Input: dimensioned drawing with shaded views. Units: mm. Origin: part minimum x, y, z. Give positions to 0.01 mm unless a question says otherwise; leave off trailing zeros. Loops run counter-clockwise (first coordinate to the right, second up) from the corner with the lowest first, then second, coordinate; pieces in that order, holes last.
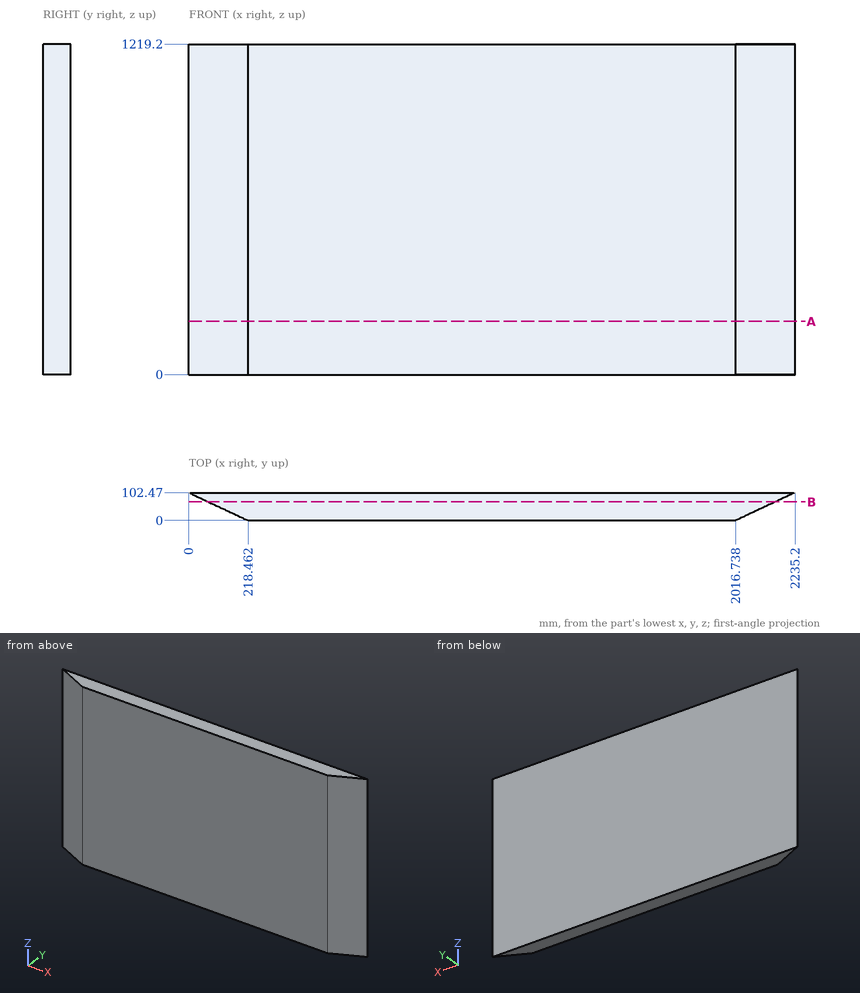
Item 1: Section query B-B on y = 68.5. Return loops of the section in (x, z).
Values follow:
outline: (72.42, 0) - (2162.78, 0) - (2162.78, 1219.2) - (72.42, 1219.2) - close
Item 2: Ray query, probe 1 along X at (y, z) = (5, 685); probe 2 along X at (y, z) = (37, 176); probe 3 along Y at (x, z) = (2031, 446.5). Return the intervals inside material, ascending.
Values follow:
probe 1: x = 207.8 to 2027.4
probe 2: x = 139.58 to 2095.62
probe 3: y = 6.69 to 102.47
Item 3: Pin query (flat end, axial travel): pin 1 (3 mm diameter, centred on y = 59, z = 766, fed in from -X); pin 2 (1 mm diameter, centred on y = 31, z = 454.5, fed in from -X) (1 decimal); pin 3 (3 mm diameter, centred on y = 42.5, z = 693.5, fed in from -X) (1 decimal). Return the tip coordinate at first contact, or that it passes through.
Values follow:
pin 1: stops at x = 89.48
pin 2: stops at x = 151.3
pin 3: stops at x = 124.7
Item 4: Section query A-A on z = 196.5. Return loops of the section in (x, y), plus the area to 3 significant figures.
Values follow:
outline: (0, 102.47) - (218.46, 0) - (2016.74, 0) - (2235.2, 102.47) - close
area: 207,000 mm2
